Check sheet for the modelled part. Datum: model origin and axes. Units: mm. A direction names the side the tool comes from. Give positions to 0.01 mm unless a question says otherwise; leave off trailing zeros. Order: outer loops, then holes, each group sorted by start corner. A loop starts at its lowest first (then second) coordinate and runs counter-clockwise, first axis right, second up.
Autodesk Inventor part; units mm, degrees
ref_plane "YZ Plane" through (0, 0, 0) normal (1, 0, 0) x (0, 1, 0)
ref_plane "XZ Plane" through (0, 0, 0) normal (0, 1, 0) x (-1, 0, 0)
ref_plane "XY Plane" through (0, 0, 0) normal (0, 0, 1) x (1, 0, 0)
sketch "Sketch1" plane through (0, 0, 0) normal (0, 0, 1) x (1, 0, 0)
  line L0 (0, 0) -> (0, 25.4)
  line L1 (0, 0) -> (0, -6.35)
  line L2 (0, 25.4) -> (0, 38.1)
  line L3 (8.4667, 25.4) -> (8.4667, 38.1)
  line L4 (8.4667, 38.1) -> (0, 38.1)
  line L5 (3.175, 17.0324) -> (0, 17.0324) construction
  line L6 (8.4667, 25.4) -> (6.8792, 25.4)
  line L7 (6.8792, 25.4) -> (0, 25.4) construction
  line L8 (0, 0) -> (3.175, 0) construction
  line L9 (3.175, 0) -> (17.91, 0) construction
  line L10 (22.6258, 3.4297) -> (23.8125, 10.16)
  line L11 (23.8125, 10.16) -> (23.8125, 13.335)
  line L12 (15.3458, 10.16) -> (6.8792, 10.16)
  line L13 (19.1558, 13.335) -> (23.8125, 13.335)
  line L14 (0, -6.35) -> (3.175, -4.2333)
  line L15 (3.175, -4.2333) -> (3.175, 0)
  line L16 (15.3458, 10.16) -> (19.1558, 13.335)
  line L17 (3.175, 0) -> (22.6258, 3.4297)
  line L18 (6.8792, 25.4) -> (6.8792, 10.16)
  dimension "d5" = 44.45
  dimension "d6" = 12.7
  dimension "d7" = 8.4667
  dimension "d12" = 2.1167
  dimension "d13" = 3.175
  dimension "d15" = 4.2333
  dimension "d18" = 3.175
  dimension "d20" = 3.175
  dimension "d21" = 3.81
  dimension "d23" = 10.16
  dimension "d24" = 10
  dimension "d26" = 23.8125
  dimension "d27" = 110
  dimension "d28" = 1.5875
  dimension "d29" = 8.4667
revolve "Revolution1" add sketch "Sketch1" angle 360 about axis through (0, 25.4, 0) along (0, -1, 0)
properties part number "Top1"
1) Material ranges on L1, parallel to Z at x = 10.5, y = 12; L2, parallel to Z at x = 9.5, y = 11; L3, parallel to Z at x = -17.5, y = 7, recorded low to high.
Recorded:
L1: z = -21.37 to -14.07, 14.07 to 21.37
L2: z = -21.84 to -13.31, 13.31 to 21.84
L3: z = -15.32 to 15.32
2) Set-up check for faces 1 (the face through (-0.69, -2.09, 3.1)), 2 (the face through (-1, 25.4, 7)), 3 (the face through (-6.72, 31.84, 5.15)): record each of +Z, -Z, +X, -X, +Y, -Y from which the full face is reachable in a straight line by a thin tool's end or side.
Recorded:
face 1: -Y
face 2: none
face 3: +Y
3) Section check A-A, the plane y = 33. Record the cut outline in (x, z).
Recorded:
outline: circle Ø16.93 at (0, 0)
4) Depth check by flat-ended pin: pin 1 Ø3 at (y, z) = (25, -5) entering from +X; pin 2 Ø5 at (x, z) = (5.5, -14) entering from -Y; pin 3 Ø12 at (x, y) = (-2, 1) entering from +Z. Enter the tip coordinate at first touch or a pass-through.
Recorded:
pin 1: stops at x = 7.68
pin 2: stops at y = 1.65
pin 3: stops at z = 23.22
5) Draft check along X on faces 4 (the face through (7, 10.16, -3)), 5 (the face through (0, 38.1, 0)), 6 (the face through (-18.897, 11.77, 14.49)), 7 (the face through (-11.49, 10.36, -10.53)). Enter one of: +X half, -X half, draft (parallel to the pull), parting line (faces both ways), or undercut.
Recorded:
face 4: undercut
face 5: draft
face 6: parting line
face 7: undercut
6) Section check B-B, the plane y = 24. Record the cut outline in (x, z), then the cut area to 3 significant figures.
Recorded:
outline: circle Ø13.76 at (0, 0)
area: 149 mm2
